Part model, mm, in its own coordinate system. Face numbers are marked on the shaded views. A direction names the side the tool comes from. Give positions to 0.01 mm unless a question says otherwise; leave off trailing zeros. Write each loop counter-clockwise with the first axis right and the second up, starting at its lowest first coordinate (ties: lowest second). Pieces come first, ordered by that corner, then holes. Notation, with made-up numbers: M -6,54.5 L 49,54.5 A26 ccw 49,86.5 Z; hole C 59,76.25 d10. An arc over 180 degrees is marked long. Answer as CSV lines item,"result". Start each with the question number.
1) Tool access for the marked faces 1 and 2: list every direction of +Z, -Z, +X, -X, +Y, -Y with a clear straight run to the whole face (end or side of a thin tool).
2) Pin check, flat tips, straight feed: pin 1 Ø3 at (y, z) = (8.5, 27.5) entering from +X; pin 2 Ø1.5 at (x, z) = (-14.5, 19.5) entering from -Y; pin 3 Ø1.5 at (y, z) = (-6.5, 29.5) entering from -X. Stop position of each tip, or through.
3) Slice it at A-A, the plane x = 0. Give the cut face in (y, z), plus the area to 3 significant figures.
4) Slice it at C-C, the plane z = 46. Give the cut face in (x, y).
5) Slice it at D-D, the plane y = -9. Give the cut face in (x, z).
6) Wall check: line 1 along Z through (x, y) = (-15, 5.5); line 2 along Z through (x, y) = (-26, -2.5); line 3 along X through (y, z) = (6, 3). Give the ranges that are in metal, low to high. Write a range as from..to.
```python
from build123d import *

# Parameters (mm, degrees)
F0_R     = 32.031836
F0_R_2   = 21.104054
F1_DEPTH = 12.7
F0_R_3   = 10.939518
F2_DEPTH = 25.4
F0_R_4   = 5.553699
F3_DEPTH = 38.1
F4_DEPTH = 50.8


with BuildPart() as f1:
    # F0 (on Top) → F1 (new body)
    with BuildSketch(Plane.XY):
        Circle(F0_R)
        Circle(F0_R_2, mode=Mode.SUBTRACT)
    extrude(amount=F1_DEPTH)

    # F0 (on Top) → F2 (join)
    with BuildSketch(Plane.XY):
        Circle(F0_R_2)
        Circle(F0_R_3, mode=Mode.SUBTRACT)
    extrude(amount=F2_DEPTH)

    # F0 (on Top) → F3 (join)
    with BuildSketch(Plane.XY):
        Circle(F0_R_3)
        Circle(F0_R_4, mode=Mode.SUBTRACT)
    extrude(amount=F3_DEPTH)

    # F0 (on Top) → F4 (join)
    with BuildSketch(Plane.XY):
        Circle(F0_R_4)
    extrude(amount=F4_DEPTH)


solid = f1.part
```
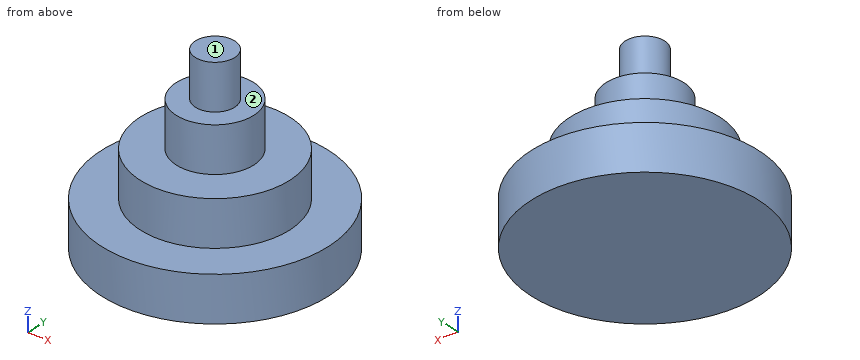
Found:
1,face 1,"+Z, +X, -X, +Y, -Y"
1,face 2,"+Z"
2,pin 1,"x = 8.41"
2,pin 2,"y = -16.01"
2,pin 3,"x = -9.31"
3,outline,"M -32.03,0 L 32.03,0 L 32.03,12.7 L 21.1,12.7 L 21.1,25.4 L 10.94,25.4 L 10.94,38.1 L 5.55,38.1 L 5.55,50.8 L -5.55,50.8 L -5.55,38.1 L -10.94,38.1 L -10.94,25.4 L -21.1,25.4 L -21.1,12.7 L -32.03,12.7 Z"
3,area,"1,770 mm²"
4,outline,"C 0,0 d11.11"
5,outline,"M -30.74,0 L 30.74,0 L 30.74,12.7 L 19.09,12.7 L 19.09,25.4 L 6.22,25.4 L 6.22,38.1 L -6.22,38.1 L -6.22,25.4 L -19.09,25.4 L -19.09,12.7 L -30.74,12.7 Z"
6,line 1,"0..25.4"
6,line 2,"0..12.7"
6,line 3,"-31.46..31.46"
